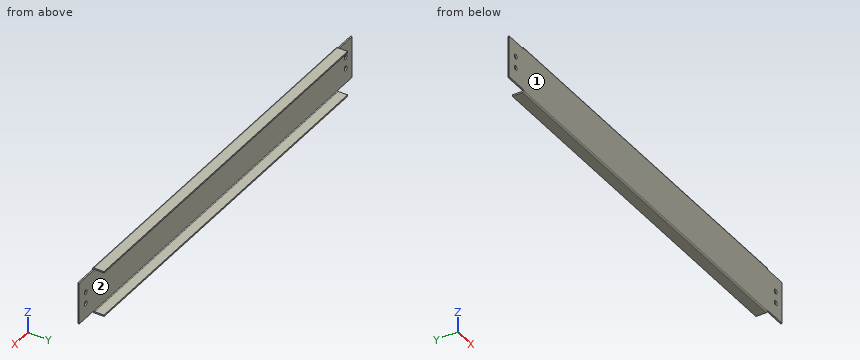
from build123d import *

# Parameters (mm, degrees)
BOSS_EXTRUDE1_DEPTH   = 210.82
SKETCH2_W             = 46.0375
SKETCH2_H             = 1.5875
BOSS_EXTRUDE2_DEPTH   = 25.4
SKETCH3_R             = 0.635
CUT_EXTRUDE1_DEPTH    = 238.841409465
F_8_CLEARANCE_HOLE1_D = 4.9149


with BuildPart() as part:
    # Sketch1 → Boss-Extrude1 (new body)
    with BuildSketch(Plane(origin=(0, 0, 0), x_dir=(0, 0, -1), z_dir=(1, 0, 0))):
        with BuildLine():
            Line((-23.8125, 0), (23.8125, 0))
            ThreePointArc((23.8125, 0), (24.935032015, 0.464967985), (25.4, 1.5875))
            Line((25.4, 1.5875), (25.4, 12.7))
            Line((25.4, 12.7), (23.8125, 12.7))
            Line((23.8125, 12.7), (23.8125, 2.38125))
            ThreePointArc((23.8125, 2.38125), (23.580016008, 1.819983992), (23.01875, 1.5875))
            Line((23.01875, 1.5875), (-23.01875, 1.5875))
            ThreePointArc((-23.01875, 1.5875), (-23.580016008, 1.819983992), (-23.8125, 2.38125))
            Line((-23.8125, 2.38125), (-23.8125, 12.7))
            Line((-23.8125, 12.7), (-25.4, 12.7))
            Line((-25.4, 12.7), (-25.4, 1.5875))
            ThreePointArc((-25.4, 1.5875), (-24.935032015, 0.464967985), (-23.8125, 0))
        make_face()
    boss_extrude1 = extrude(amount=BOSS_EXTRUDE1_DEPTH)

    # Sketch2 → Boss-Extrude2 (add)
    with BuildSketch(Plane(origin=(210.82, 0, 0), x_dir=(0, 0, -1), z_dir=(1, 0, 0))):
        with Locations((0, 0.79375)):
            Rectangle(SKETCH2_W, SKETCH2_H)
    boss_extrude2 = extrude(amount=BOSS_EXTRUDE2_DEPTH)

    # Mirror1: Boss-Extrude1, Boss-Extrude2 across plane
    add(boss_extrude1.mirror(Plane(origin=(0, 0, 0), x_dir=(0, 0, 1), z_dir=(1, 0, 0))))
    add(boss_extrude2.mirror(Plane(origin=(0, 0, 0), x_dir=(0, 0, 1), z_dir=(1, 0, 0))))

    # Sketch3 → Cut-Extrude1 (cut, through all)
    with BuildSketch(Plane(origin=(0, 1.5875, 0), x_dir=(1, 0, 0), z_dir=(0, 1, 0))):
        with Locations(Location((225.044, -6.35, 0), (0, 0, 270))):
            Circle(SKETCH3_R)
        with Locations(Location((225.044, 6.35, 0), (0, 0, 270))):
            Circle(SKETCH3_R)
    extrude(amount=-CUT_EXTRUDE1_DEPTH, mode=Mode.SUBTRACT)

    # #8 Clearance Hole1 (through all)
    with Locations(Plane(origin=(0, 1.5875, 0), x_dir=(1, 0, 0), z_dir=(0, 1, 0))):
        with Locations((225.044, -6.35), (225.044, 6.35)):
            f_8_clearance_hole1 = Hole(F_8_CLEARANCE_HOLE1_D / 2)

    # Mirror2: #8 Clearance Hole1 across plane
    add(f_8_clearance_hole1.mirror(Plane(origin=(0, 0, 0), x_dir=(0, 0, 1), z_dir=(1, 0, 0))), mode=Mode.SUBTRACT)


solid = part.part
For this review, take the finished solid that the model builds, in its own axes (mm). Face numbers are marked on the shaded views. Give positions to 0.01 mm unless a question says otherwise; leave off trailing zeros. Order: outer loops, then holes, each group sorted by start corner. A loop starts at its lowest first (then second) coordinate and runs counter-clockwise, first axis right, second up. Notation, with made-up numbers: M 80.5,14.25 L 92.5,14.25 A19 cw 92.5,25.25 Z; hole C 29,-23 d6. An arc over 180 degrees is marked long. Answer in a Markdown table with one row per item. Add a question column.
(1) Wall thickness on probe 1 along Z at (x, y) = (118.5, 5.5); probe 2 along Y at (x, z) = (-26, 8); probe 3 along Z at (x, y) = (128, 1.25): over which ranges is each line inside the solid? List them lowest first. Write a range as [from, to].
(2) For pin 1 (0.8 mm diameter, centred on x = -218.5, y = 1, fed in from +Z); pin 2 (8 mm diameter, centred on x = 20.5, z = 4, fed in from +Y); pin 3 (1.2 mm diameter, centred on y = 8.5, z = -24.5, fed in from -X); pin 4 (4.5 mm diameter, centred on x = 225.044, z = 6.35, fed in from -Y), all flat-tipped, find the tip position at first contact; note any pin that passes through.
(3) Consider section B-B on z = 16.5. State the section outline as (x, y) points, and give its area (3 significant figures).
(4) Consider section A-A on x = 119. State the section outline as (y, z) points (1 decimal), and give its area (3 significant figures).
(5) Mouldability with a two-part tool opening along Z and no side actions: class the marked faces 1 and 2 as +Z half, -Z half, draft (parallel to the pull), parting line (faces both ways), or undercut.
Evaluation:
| question | item | result |
|---|---|---|
| 1 | probe 1 | z = [-25.4, -23.81], [23.81, 25.4] |
| 1 | probe 2 | y = [0, 1.59] |
| 1 | probe 3 | z = [-25.36, 25.36] |
| 2 | pin 1 | stops at z = 23.02 |
| 2 | pin 2 | stops at y = 1.59 |
| 2 | pin 3 | stops at x = -210.82 |
| 2 | pin 4 | passes through |
| 3 | outline | M -236.22,0 L 236.22,0 L 236.22,1.59 L -236.22,1.59 Z |
| 3 | area | 750 mm^2 |
| 4 | outline | M 0,-23.8 A1.6 ccw 1.6,-25.4 L 12.7,-25.4 L 12.7,-23.8 L 2.4,-23.8 A0.8 cw 1.6,-23 L 1.6,23 A0.8 cw 2.4,23.8 L 12.7,23.8 L 12.7,25.4 L 1.6,25.4 A1.6 ccw 0,23.8 Z |
| 4 | area | 115 mm^2 |
| 5 | face 1 | draft |
| 5 | face 2 | undercut |
